The model under review builds one solid part; all positions refer to its coordinate system, in mm. A direction names the side the tool comes from. Coordinates: 2 decimals unless noted, no trailing zeros. Write each loop counter-clockwise with the first axis right and the second up, starting at its lowest first coordinate (ties: lowest second). Pieces come first, ordered by that corner, then holes. Notation, with made-up numbers: M 20,-39.5 L 78,-39.5 A24 cw 78,-11.5 Z; hole C 52.25,-28 d2. An arc over 180 degrees is marked long. Answer as a JSON object with one key per item and string values.
```python
from build123d import *

# Parameters (mm, degrees)
CROQUIS1_R                 = 7.95
SALIENTE_EXTRUIR1_DEPTH    = 7.5
CROQUIS2_R                 = 8.45
SALIENTE_EXTRUIR2_DEPTH    = 0.5
SALIENTE_EXTRUIR3_START    = -14.5
CROQUIS2_2_R               = 8.45
SALIENTE_EXTRUIR3_DEPTH    = 0.5
CROQUIS3_R                 = 5
SALIENTE_EXTRUIR4_DEPTH    = 21
CORTAR_EXTRUIR1_DEPTH      = 24.728779994
CORTAR_EXTRUIR1_DEPTH_BACK = 24.728779994
CROQUIS4_R                 = 3
CROQUIS10_R                = 4
CORTAR_EXTRUIR2_DEPTH      = 25.162057032


with BuildPart() as part:
    # Croquis1 → Saliente-Extruir1 (new, symmetric)
    with BuildSketch(Plane(origin=(0, 0, 0), x_dir=(-1, 0, 0), z_dir=(0, 1, 0))):
        with Locations(Location((0, 0, 0), (0, 0, 90))):
            Circle(CROQUIS1_R)
    extrude(amount=SALIENTE_EXTRUIR1_DEPTH, both=True)

    # Croquis2 → Saliente-Extruir2 (add)
    with BuildSketch(Plane(origin=(0, 7.5, 0), x_dir=(-1, 0, 0), z_dir=(0, 1, 0))):
        with Locations(Location((0, 0, 0), (0, 0, 90))):
            Circle(CROQUIS2_R)
    extrude(amount=-SALIENTE_EXTRUIR2_DEPTH)

    # Croquis2<2> → Saliente-Extruir3 (add)
    with BuildSketch(Plane(origin=(0, 7.5, 0), x_dir=(-1, 0, 0), z_dir=(0, 1, 0)).offset(SALIENTE_EXTRUIR3_START)):
        with Locations(Location((0, 0, 0), (0, 0, 90))):
            Circle(CROQUIS2_2_R)
    extrude(amount=-SALIENTE_EXTRUIR3_DEPTH)

    # Croquis3 → Saliente-Extruir4 (add)
    with BuildSketch(Plane(origin=(0, -7.5, 0), x_dir=(-1, 0, 0), z_dir=(0, 1, 0))):
        with Locations(Location((0, 0, 0), (0, 0, 270))):
            Circle(CROQUIS3_R)
    extrude(amount=SALIENTE_EXTRUIR4_DEPTH)

    # Croquis4 → Cortar-Extruir1 (cut, two sides: drawn at the far end of the back side and taken through both)
    with BuildSketch(Plane(origin=(0, -7, 0), x_dir=(-1, 0, 0), z_dir=(0, 1, 0)).offset(-CORTAR_EXTRUIR1_DEPTH_BACK)):
        with Locations(Location((0, 0, 0), (0, 0, 90))):
            Circle(CROQUIS4_R)
    extrude(amount=CORTAR_EXTRUIR1_DEPTH + CORTAR_EXTRUIR1_DEPTH_BACK, mode=Mode.SUBTRACT)

    # Croquis10 → Cortar-Extruir2 (cut, through all)
    with BuildSketch(Plane.XZ.offset(7.5)):
        with Locations(Location((0, 0, 0), (0, 0, 270))):
            Circle(CROQUIS10_R)
    extrude(amount=-CORTAR_EXTRUIR2_DEPTH, mode=Mode.SUBTRACT)


solid = part.part
```
(1) Draft analysis for pull direction Y (two halves, no side actions). For faces 4 (the face through (2, -7.5, -4)), 5 (the face through (2.54, 7.25, 8.06)), 6 (the face through (-3.1, 7, 7.5)), 7 (the face through (-4, 7.5, 4)), state which applies: released by +Y, released by -Y, zero draft, split by the parting line, or undercut.
Results list:
{"face 4": "released by -Y", "face 5": "zero draft", "face 6": "undercut", "face 7": "released by +Y"}
(2) Add section D-D on x = 6. Give the boundary of the cut face in (y, z), and give its area (3 significant figures).
Results list:
{"outline": "M -7.5,-5.95 L -7,-5.95 L -7,-5.22 L 7,-5.22 L 7,-5.95 L 7.5,-5.95 L 7.5,5.95 L 7,5.95 L 7,5.22 L -7,5.22 L -7,5.95 L -7.5,5.95 Z", "area": "158 mm²"}
(3) For faces 1 (the face through (-4.837, 0.098, -6.309)), 2 (the face through (4.88, 10.46, 1.08)), 3 (the face through (-3.905, 2.853, 0.867)), list the 3-axis set-ups (+Z, -Z, +X, -X, +Y, -Y) from which the entire face can be reached by the end or side of a thin tool; tool diameter is ignored.
Results list:
{"face 1": "none", "face 2": "+Y", "face 3": "+Y, -Y"}
(4) Wall thickness on line 1 along Y through (x, z) = (3.5, -7.5); line 2 along X through (y, z) = (0.5, 0); line 3 along Y through (x, z) = (5.5, 2.25): over which ranges is each line inside the solid? List them lowest first. Write a range as from..to.
Results list:
{"line 1": "-7.5..-7, 7..7.5", "line 2": "-7.95..-4, 4..7.95", "line 3": "-7.5..7.5"}
(5) For pin 1 Ø1.5 at (y, z) = (0, 4) entering from +X; pin 2 Ø3 at (x, y) = (5, 6.5) entering from -Z; pin 3 Ø1.5 at (y, z) = (7.5, 1) entering from +X; pin 4 Ø5 at (x, z) = (1.5, -2.5) entering from +Y, all flat-tipped, find the tip position at first contact; note any pin that passes through.
Results list:
{"pin 1": "x = 7.26", "pin 2": "z = -7.65", "pin 3": "x = 8.45", "pin 4": "y = 13.5"}
(6) Add section B-B on x = 0. Give the boundary of the cut face in (y, z), and give its area (4 significant figures).
Results list:
{"outline": "M -7.5,-8.45 L -7,-8.45 L -7,-7.95 L 7,-7.95 L 7,-8.45 L 7.5,-8.45 L 7.5,-5 L 13.5,-5 L 13.5,-4 L -7.5,-4 Z; M -7.5,4 L 13.5,4 L 13.5,5 L 7.5,5 L 7.5,8.45 L 7,8.45 L 7,7.95 L -7,7.95 L -7,8.45 L -7.5,8.45 Z", "area": "131.5 mm²"}
(7) Add section A-A on z = 0. Give the boundary of the cut face in (x, y).
Results list:
{"outline": "M -8.45,-7.5 L -4,-7.5 L -4,13.5 L -5,13.5 L -5,7.5 L -8.45,7.5 L -8.45,7 L -7.95,7 L -7.95,-7 L -8.45,-7 Z; M 4,-7.5 L 8.45,-7.5 L 8.45,-7 L 7.95,-7 L 7.95,7 L 8.45,7 L 8.45,7.5 L 5,7.5 L 5,13.5 L 4,13.5 Z"}
(8) Add section C-C on y = 0. Give the boundary of the cut face in (x, z).
Results list:
{"outline": "C 0,0 d15.9; hole C 0,0 d8"}
